Work out the finished part from the listing and answer in its coordinate system (mm). Face numbers are marked on the shaded views. A direction names the side the tool comes from. Give positions to 0.01 mm unless a question says otherwise; leave off trailing zeros. Loops run counter-clockwise (first coordinate to the right, second up) from the corner with the lowest first, then second, coordinate; pieces in that order, holes last. Notation, with made-up numbers: (21, 32.5) -> (76, 32.5) arc R14 cw to (76, 46.5) -> close; hole circle Ø11 at (6.5, 10). An arc over 180 degrees is marked (long way). Answer as CSV lines item,"result". Start each with the question number.
1. Determine the mould class of the marked faces 1, 2 and 3 for opening direction Z: +Z half, -Z half, draft (parallel to the pull), parting line (faces both ways), or undercut.
2. Find section B-B, the plane z = 2.25. Give the vertices of the cut face in (x, y), and give its area (3 significant figures).
3. Find section C-C, the plane y = 9. Give the vertices of the cut face in (x, z), and give its area (3 significant figures).
4. A tool of negligible diameter and unlimited length cuts with its end or side. For the marked faces 4, 5, 6, 7 and 8, from which of +Z, -Z, +X, -X, +Y, -Y can it reach the whole face along a straight path? Write none if from no direction.
5. Find section A-A, the plane x = -3.25. Give the vertices of the cut face in (y, z), and give its area (3 significant figures).
6. Find section D-D, the plane x = 0.75. Give the vertices of the cut face in (y, z).
7. Find the intervals of material crossed by line 1 along Y through (x, z) = (2.25, -3.75); line 2 along Y through (x, z) = (-4.5, 4.5); line 3 along Z through (x, y) = (-2.75, 3), in increasing order.
8. Flat-ended cylindrical pins translate along their axes: pin 1 Ø2.5 at (x, y) = (2, 11.5) entering from -Z; pin 2 Ø1 at (y, z) = (7, -3) entering from -X; pin 3 Ø4 at (x, y) = (-2, 8.5) entering from +Z. Find the tip coordinate at first contact, or state that the pin passes through.
from build123d import *

# Parameters (mm, degrees)
SKETCH_1_W          = 12
SKETCH_1_H          = 10
EXTRUDE_1_DEPTH     = 24
FILLET_1_R          = 1
SKETCH_2_OUTSIDE_W  = 19.728
SKETCH_2_OUTSIDE_H  = 17.728
CUT_EXTRUDE_1_DEPTH = 16
SKETCH_3_R          = 1.5
EXTRUDE_2_DEPTH     = 13


with BuildPart() as part:
    # 草图1 → 凸台-拉伸1 (new body)
    with BuildSketch(Plane(origin=(0, 0, 0), x_dir=(1, 0, 0), z_dir=(0, 1, 0))):
        Rectangle(SKETCH_1_W, SKETCH_1_H)
    extrude(amount=EXTRUDE_1_DEPTH)

    # 圆角1
    fillet_1_edges = [part.edges().sort_by_distance(p)[0] for p in [
        (6, 12, 5),
        (-6, 12, 5),
        (-6, 12, -5),
        (6, 12, -5),
    ]]
    fillet(fillet_1_edges, radius=FILLET_1_R)

    # 草图2 outside → 切除-拉伸1 (cut)
    with BuildSketch(Plane.XZ):
        Rectangle(SKETCH_2_OUTSIDE_W, SKETCH_2_OUTSIDE_H)
        with BuildLine():
            Line((-3.968626967, -4.5), (3.968626967, -4.5))
            ThreePointArc((3.968626967, -4.5), (5.468626967, -2.468626967), (6, 0))
            ThreePointArc((6, 0), (5.468626967, 2.468626967), (3.968626967, 4.5))
            Line((3.968626967, 4.5), (-3.968626967, 4.5))
            ThreePointArc((-3.968626967, 4.5), (-5.468626967, 2.468626967), (-6, 0))
            ThreePointArc((-6, 0), (-5.468626967, -2.468626967), (-3.968626967, -4.5))
        make_face(mode=Mode.SUBTRACT)
    extrude(amount=-CUT_EXTRUDE_1_DEPTH, mode=Mode.SUBTRACT)

    # 草图3 → 凸台-拉伸2 (add)
    with BuildSketch(Plane(origin=(0, 24, 0), x_dir=(1, 0, 0), z_dir=(0, 1, 0))):
        with Locations(Location((0, 0, 0), (0, 0, 90))):
            Circle(SKETCH_3_R)
    extrude(amount=EXTRUDE_2_DEPTH)


solid = part.part
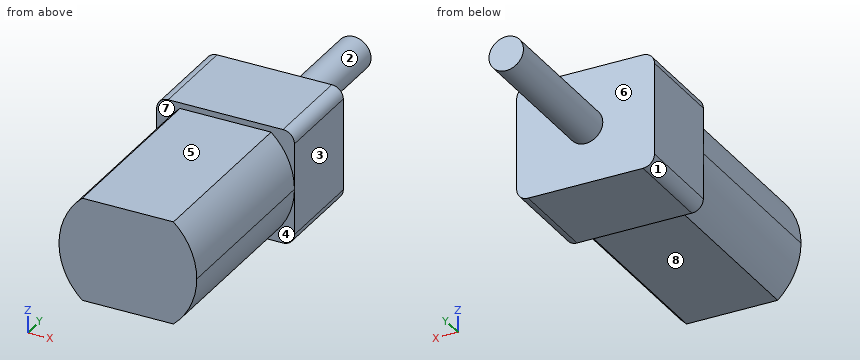
Resolved:
1,face 1,"-Z half"
1,face 2,"parting line"
1,face 3,"draft"
2,outline,"(-6, 16) -> (-5.56, 16) -> (-5.56, 0) -> (5.56, 0) -> (5.56, 16) -> (6, 16) -> (6, 24) -> (-6, 24) -> close"
2,area,"274 mm^2"
3,outline,"(-3.97, -4.5) -> (3.97, -4.5) arc R6 ccw to (3.97, 4.5) -> (-3.97, 4.5) arc R6 ccw to start"
3,area,"96.8 mm^2"
4,face 4,"-Z, -Y"
4,face 5,"+Z, +X, -X, -Y"
4,face 6,"+Y"
4,face 7,"+Z, -Y"
4,face 8,"-Z, +X, -X, -Y"
5,outline,"(0, -4.5) -> (16, -4.5) -> (16, -5) -> (24, -5) -> (24, 5) -> (16, 5) -> (16, 4.5) -> (0, 4.5) -> close"
5,area,"224 mm^2"
6,outline,"(0, -4.5) -> (16, -4.5) -> (16, -5) -> (24, -5) -> (24, -1.3) -> (37, -1.3) -> (37, 1.3) -> (24, 1.3) -> (24, 5) -> (16, 5) -> (16, 4.5) -> (0, 4.5) -> close"
7,line 1,"y = 0 to 24"
7,line 2,"y = 16 to 24"
7,line 3,"z = -4.5 to 4.5"
8,pin 1,"stops at z = -4.5"
8,pin 2,"stops at x = -5.45"
8,pin 3,"stops at z = 4.5"
